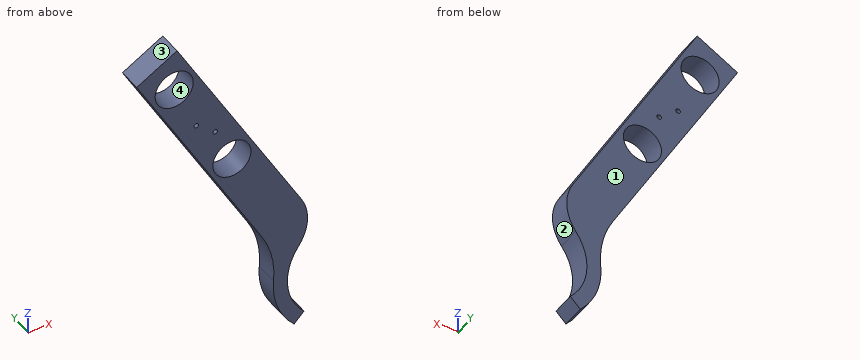
from build123d import *

# Parameters (mm, degrees)
SKETCH_2_R          = 4.1
EXTRUDE_1_DEPTH     = 5
FILLET_1_R          = 20
SKETCH_6_R          = 0.5
CUT_EXTRUDE_3_DEPTH = 51.047278583
FILLET_2_R          = 10


with BuildPart() as part:
    # ｽｹｯﾁ2 → ﾎﾞｽ - 押し出し1 (new body)
    with BuildSketch(Plane(origin=(0, 0, 0), x_dir=(1, 0, 0), z_dir=(0, 1, 0))):
        with BuildLine():
            Line((10.525449769, 28.464000424), (-20.21962407, -25.270887679))
            Line((-20.21962407, -25.270887679), (-11.539937113, -30.237076794))
            Line((-11.539937113, -30.237076794), (19.283832312, 23.635351995))
            ThreePointArc((19.283832312, 23.635351995), (12.394035574, 32.590650485), (15.787121591, 43.368110179))
            Line((15.787121591, 43.368110179), (13.648123578, 45.507108192))
            ThreePointArc((13.648123578, 45.507108192), (9.431206098, 37.472115328), (10.525449769, 28.464000424))
        make_face()
        with Locations(Location((-12.155138755, -21.244217019, 0), (0, 0, 270))):
            Circle(SKETCH_2_R, mode=Mode.SUBTRACT)
        with Locations(Location((0.260334032, 0.455000374, 0), (0, 0, 270))):
            Circle(SKETCH_2_R, mode=Mode.SUBTRACT)
    extrude(amount=EXTRUDE_1_DEPTH)

    # ﾌｨﾚｯﾄ1
    fillet_1_edges = [part.edges().sort_by_distance(p)[0] for p in [
        (10.525449769, 2.5, -28.464000424),
    ]]
    fillet(fillet_1_edges, radius=FILLET_1_R)

    # ｽｹｯﾁ6 → ｶｯﾄ - 押し出し3 (cut, through all)
    with BuildSketch(Plane(origin=(0, 5, 0), x_dir=(1, 0, 0), z_dir=(0, 1, 0))):
        with Locations(Location((-7.408738509, -10.639307665, 0), (0, 0, 270))):
            Circle(SKETCH_6_R)
        with Locations(Location((-3.329499593, -7.444424173, 0), (0, 0, 270))):
            Circle(SKETCH_6_R)
    extrude(amount=-CUT_EXTRUDE_3_DEPTH, mode=Mode.SUBTRACT)

    # ﾌｨﾚｯﾄ2
    fillet_2_edges = [part.edges().sort_by_distance(p)[0] for p in [
        (19.283832312, 2.5, -23.635351995),
    ]]
    fillet(fillet_2_edges, radius=FILLET_2_R)


solid = part.part
Verification items for the finished model (mm, model axes). Face numbers are marked on the shaded views. Coordinates: 2 decimals unless noted, no trailing zeros. Order: outer loops, then holes, each group sorted by start corner. A loop starts at its lowest first (then second) coordinate and runs counter-clockwise, first axis right, second up. Notation, with made-up numbers: M 13.5,-6.75 L 24.5,-6.75 A25 cw 24.5,29.25 Z; hole C -6.75,85.5 d7. An arc over 180 degrees is marked long. Return JSON: item names as keys, results as strings.
1) Cross-section at A-A, the plane z = 1. Record the boundary of the cut face in (x, y), and give its area (3 significant figures).
Answer list:
{"outline": "M -6.33,0 L -3.57,0 L -3.57,5 L -6.33,5 Z; M 4.09,0 L 5.19,0 L 5.19,5 L 4.09,5 Z", "area": "19.3 mm2"}
2) Cross-section at D-D, the plane z = -9. Record the boundary of the cut face in (x, y), and give its area (3 significant figures).
Answer list:
{"outline": "M -0.61,0 L 10.91,0 L 10.91,5 L -0.61,5 Z", "area": "57.6 mm2"}
3) Gauge pin test, flat ends, axial feed: pin 1 (1.5 mm diameter, centred on y = 3.5, z = -4.5, fed in from +X); pin 2 (2 mm diameter, centred on y = 1.5, z = 11, fed in from -X); pin 3 (1 mm diameter, centred on y = 1.5, z = 1.5, fed in from +X). Record the tip position at first contact, or that the pin passes through.
Answer list:
{"pin 1": "x = 8.76", "pin 2": "x = -12.63", "pin 3": "x = 5.19"}
4) Release check for a two-part mould opening along X. For the marked faces 1, 2, 3 and 4 record: +X half, -X half, draft (parallel to the pull), parting line (faces both ways), or undercut.
Answer list:
{"face 1": "draft", "face 2": "+X half", "face 3": "-X half", "face 4": "undercut"}
5) Thickness scan on L1, parallel to Z at x = -2, y = 2.75; L2, parallel to X at y = 4.6, z = -34.5; L3, parallel to X at y = 1.3, z = 21. Record the ranges inside material, lowest first. Write a range as [from, to].
Answer list:
{"L1": "[-6.57, -3.88], [2.97, 13.56]", "L2": "[9.18, 12.21]", "L3": "[-17.78, -16.25], [-8.06, -6.25]"}
6) Cross-section at B-B, the plane x = -14.5. Record the boundary of the cut face in (y, z).
Answer list:
{"outline": "M 0,15.27 L 5,15.27 L 5,17.88 L 0,17.88 Z; M 0,24.61 L 5,24.61 L 5,28.54 L 0,28.54 Z"}
7) Cross-section at C-C, the plane y = 0.85. Count the separate pieces of the cut face and the enclosed holes in it, and give its area (3 significant figures).
Answer list:
{"separate pieces": "1", "enclosed holes": "4", "area": "566 mm2"}
